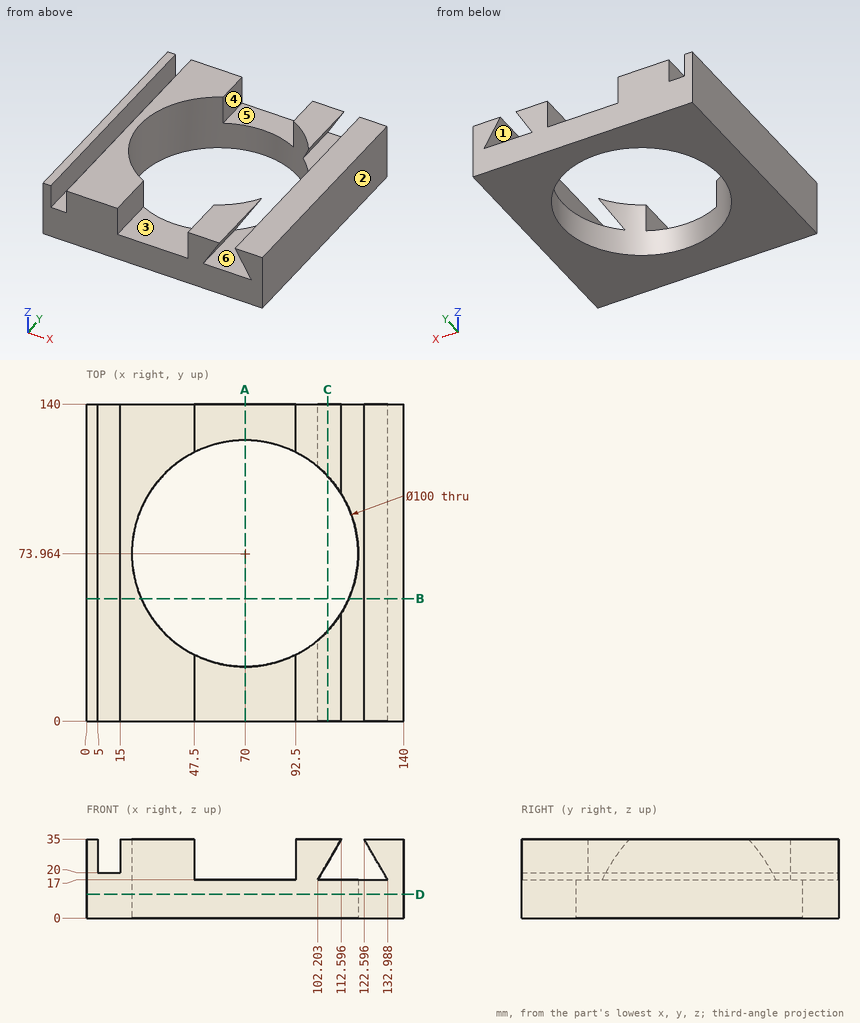
Can you work these out from the drawing? Everything is in mm from the part's minimum corner. A direction names the side the tool comes from. Round coordinates to 2 decimals unless told otherwise and drop trailing zeros. Order: outer loops, then holes, each group sorted by start corner. A loop starts at its lowest first (then second) coordinate and runs counter-clockwise, first axis right, second up. Notation, with made-up numbers: (46, 37) - (104, 37) arc R11 cw to (104, 56) - close; hole circle Ø7 at (79, -18.5). An arc over 180 degrees is marked (long way). Answer in a Markdown table with one row per item.
(1) Suppose I cut it at C-C, the plane x = 106.5. Please give me the cut outline in (y, z), plus the area to 3 significant figures.
From the geometry:
| item | result |
|---|---|
| outline | (0, 0) - (39.79, 0) - (39.79, 17) - (0, 17) - close; (0, 24.44) - (39.79, 24.44) - (39.79, 35) - (0, 35) - close; (108.14, 0) - (140, 0) - (140, 17) - (108.14, 17) - close; (108.14, 24.44) - (140, 24.44) - (140, 35) - (108.14, 35) - close |
| area | 1,970 mm2 |
(2) If we mould it in two halves opening along Z, with no side actions, what happens to the marked faces 4, 5 and 6? For each: released by +Z, released by -Z, zero draft, split by the parting line, or undercut.
From the geometry:
| item | result |
|---|---|
| face 4 | zero draft |
| face 5 | released by +Z |
| face 6 | undercut |
(3) Suppose I cut it at A-A, the plane x = 70. Please give me the cut outline in (y, z), plus the area to 3 significant figures.
From the geometry:
| item | result |
|---|---|
| outline | (0, 0) - (23.96, 0) - (23.96, 17) - (0, 17) - close; (123.96, 0) - (140, 0) - (140, 17) - (123.96, 17) - close |
| area | 680 mm2 |
(4) Please list where these lines run through material, in increasing order: L1, parallel to Y at x = 70, z = 8; L2, parallel to X at y = 64.5, z = 20.5 (1 decimal); L3, parallel to X at y = 43.5, z = 23 (1 decimal). Write a range as from..to.
From the geometry:
| item | result |
|---|---|
| L1 | y = 0..23.96, 123.96..140 |
| L2 | x = 0..5, 15..20.9, 131..140 |
| L3 | x = 0..5, 15..30.4, 129.5..140 |
(5) Suppose I cut it at B-B, the plane y = 54. Please give me the cut outline in (x, z) (1 decimal).
From the geometry:
| item | result |
|---|---|
| outline | (0, 0) - (24.2, 0) - (24.2, 35) - (15, 35) - (15, 20) - (5, 20) - (5, 35) - (0, 35) - close; (115.8, 0) - (140, 0) - (140, 35) - (122.6, 35) - (133, 17) - (115.8, 17) - close |
(6) Suppose I cut it at D-D, the plane z = 10.5. Please give me the cut outline in (x, y).
From the geometry:
| item | result |
|---|---|
| outline | (0, 0) - (140, 0) - (140, 140) - (0, 140) - close; hole circle Ø100 at (70, 73.96) |
(7) For P1, Ø10, axis at x = 115, y = 76, coming from the +Z side; P2, Ø5, axis at x = 94.5, z = 10.5, coming from the -Y side, each with a flat end and sliding along its axis, tell me the tip position at first contact or that it passes through.
From the geometry:
| item | result |
|---|---|
| P1 | stops at z = 17 |
| P2 | stops at y = 0 |
(8) Which directions (+Z, -Z, +X, -X, +Y, -Y) give clear straight access to the entire face, cutting with the end or side of a thin tool? Please do the marked faces 1, 2 and 3.
From the geometry:
| item | result |
|---|---|
| face 1 | +Y, -Y |
| face 2 | +Z, -Z, +X, +Y, -Y |
| face 3 | +Z, +Y, -Y |
